Design review of the part built by this model. Coordinates are the model's own, in mm. Face numbers are marked on the shaded views. A direction names the side the tool comes from. Give positions to 0.01 mm unless a question says otherwise; leave off trailing zeros. Order: outer loops, then holes, each group sorted by start corner. A loop starts at its lowest first (then second) coordinate and runs counter-clockwise, first axis right, second up. Notation, with made-up numbers: (69.5, 57) -> (73.5, 57) arc R32 ccw to (73.5, 83) -> close; hole circle Ø4 at (3, 42.5). An arc over 180 degrees is marked (long way). Return JSON: item names as keys, results as strings.
```python
from build123d import *

# Parameters (mm, degrees)
SKETCH1_R           = 30
BOSS_EXTRUDE1_DEPTH = 10
SKETCH2_R           = 6
CUT_EXTRUDE1_DEPTH  = 44.588989435
SKETCH3_R           = 8
CUT_EXTRUDE2_DEPTH  = 5
SKETCH4_R           = 1.75
CUT_EXTRUDE3_DEPTH  = 44.588989435
CUT_EXTRUDE4_DEPTH  = 2


with BuildPart() as part:
    # Sketch1 → Boss-Extrude1 (new body)
    with BuildSketch(Plane.XY):
        Circle(SKETCH1_R)
    extrude(amount=BOSS_EXTRUDE1_DEPTH)

    # Sketch2 → Cut-Extrude1 (cut, through all)
    with BuildSketch(Plane(origin=(0, 0, 0), x_dir=(-1, 0, 0), z_dir=(0, 0, -1))):
        Circle(SKETCH2_R)
    extrude(amount=-CUT_EXTRUDE1_DEPTH, mode=Mode.SUBTRACT)

    # Sketch3 → Cut-Extrude2 (cut)
    with BuildSketch(Plane(origin=(0, 0, 0), x_dir=(-1, 0, 0), z_dir=(0, 0, -1))):
        Circle(SKETCH3_R)
    extrude(amount=-CUT_EXTRUDE2_DEPTH, mode=Mode.SUBTRACT)

    # Sketch4 → Cut-Extrude3 (cut, through all)
    with BuildSketch(Plane(origin=(0, 0, 0), x_dir=(-1, 0, 0), z_dir=(0, 0, -1))):
        with Locations((-15, 15)):
            Circle(SKETCH4_R)
        with Locations(Location((15, 15, 0), (0, 0, 180))):
            Circle(SKETCH4_R)
        with Locations((15, -15)):
            Circle(SKETCH4_R)
        with Locations(Location((-15, -15, 0), (0, 0, 180))):
            Circle(SKETCH4_R)
    extrude(amount=-CUT_EXTRUDE3_DEPTH, mode=Mode.SUBTRACT)

    # Sketch5 → Cut-Extrude4 (cut)
    with BuildSketch(Plane(origin=(0, 0, 0), x_dir=(-1, 0, 0), z_dir=(0, 0, -1))):
        Polygon((-11.709103466, 15), (-13.354551733, 17.85), (-16.645448267, 17.85), (-18.290896534, 15), (-16.645448267, 12.15), (-13.354551733, 12.15), align=None)
        Polygon((13.354551733, 12.15), (11.709103466, 15), (13.354551733, 17.85), (16.645448267, 17.85), (18.290896534, 15), (16.645448267, 12.15), align=None)
        Polygon((11.709103466, -15), (13.354551733, -17.85), (16.645448267, -17.85), (18.290896534, -15), (16.645448267, -12.15), (13.354551733, -12.15), align=None)
        Polygon((-13.354551733, -12.15), (-11.709103466, -15), (-13.354551733, -17.85), (-16.645448267, -17.85), (-18.290896534, -15), (-16.645448267, -12.15), align=None)
    extrude(amount=-CUT_EXTRUDE4_DEPTH, mode=Mode.SUBTRACT)


solid = part.part
```
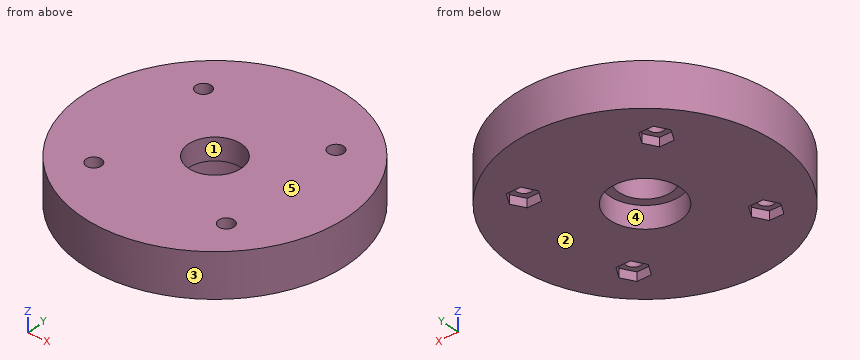
Item 1: Machinability: for the marked faces 4 and 5, which of the approach directions +Z, -Z, +X, -X, +Y, -Y give a long, thin tool a straight path to every point of the face, cutting with its end or side? Answer none if there is none.
Result set:
{"face 4": "-Z", "face 5": "+Z, +X, -X, +Y, -Y"}
Item 2: Add section D-D (x = 15). Give the boundary of the cut face in (y, z).
Result set:
{"outline": "(-25.98, 0) -> (-17.85, 0) -> (-17.85, 2) -> (-16.75, 2) -> (-16.75, 10) -> (-25.98, 10) -> close; (-13.25, 2) -> (-12.15, 2) -> (-12.15, 0) -> (12.15, 0) -> (12.15, 2) -> (13.25, 2) -> (13.25, 10) -> (-13.25, 10) -> close; (16.75, 2) -> (17.85, 2) -> (17.85, 0) -> (25.98, 0) -> (25.98, 10) -> (16.75, 10) -> close"}
Item 3: Add section B-B (z = 0.75). Give the boundary of the cut face in (x, y), plus the area to 3 significant figures.
Result set:
{"outline": "circle Ø60 at (0, 0); hole (-18.29, -15) -> (-16.65, -17.85) -> (-13.35, -17.85) -> (-11.71, -15) -> (-13.35, -12.15) -> (-16.65, -12.15) -> close; hole (-18.29, 15) -> (-16.65, 12.15) -> (-13.35, 12.15) -> (-11.71, 15) -> (-13.35, 17.85) -> (-16.65, 17.85) -> close; hole circle Ø16 at (0, 0); hole (11.71, -15) -> (13.35, -17.85) -> (16.65, -17.85) -> (18.29, -15) -> (16.65, -12.15) -> (13.35, -12.15) -> close; hole (11.71, 15) -> (13.35, 12.15) -> (16.65, 12.15) -> (18.29, 15) -> (16.65, 17.85) -> (13.35, 17.85) -> close", "area": "2,510 mm^2"}
Item 4: Add section A-A (y = 0). Give the boundary of the cut face in (x, z), plus the area to 3 significant figures.
Result set:
{"outline": "(-30, 0) -> (-8, 0) -> (-8, 5) -> (-6, 5) -> (-6, 10) -> (-30, 10) -> close; (6, 5) -> (8, 5) -> (8, 0) -> (30, 0) -> (30, 10) -> (6, 10) -> close", "area": "460 mm^2"}
Item 5: Mouldability with a two-part tool opening along X and no side actions: class the marked faces 1, 2 and 3 as released by +X, released by -X, zero draft, split by the parting line, or undercut.
Result set:
{"face 1": "undercut", "face 2": "zero draft", "face 3": "split by the parting line"}
Item 6: Wall thickness on L1, parallel to Y at x = 0, z = 1.1; L2, parallel to Y at x = 14, z = 9.25; L3, parallel to Y at x = -15, z = 8.25: over which ranges is each line inside the solid? List them lowest first. Write a range as [from, to].
Result set:
{"L1": "y = [-30, -8], [8, 30]", "L2": "y = [-26.53, -16.44], [-13.56, 13.56], [16.44, 26.53]", "L3": "y = [-25.98, -16.75], [-13.25, 13.25], [16.75, 25.98]"}
Item 7: For pin 1 (1 mm diameter, centred on x = -1.5, z = 2, fed in from +Y); pin 2 (3 mm diameter, centred on x = -15, y = 15, fed in from -Z); pin 3 (4 mm diameter, centred on x = -14, z = 6, fed in from -Y); pin 4 (6 mm diameter, centred on y = 8.5, z = 4.5, fed in from -X), all flat-tipped, find the tip position at first contact; note any pin that passes through.
Result set:
{"pin 1": "stops at y = 29.98", "pin 2": "passes through", "pin 3": "stops at y = -27.5", "pin 4": "stops at x = -29.49"}
